Build history of the part. All positions in model axes, mm. Face numbers are marked on the shaded views. Give positions to 0.01 mm unless a question says otherwise; leave off trailing zeros. Order: outer loops, then holes, each group sorted by start corner. A loop starts at its lowest first (then second) coordinate and runs counter-clockwise, first axis right, second up. Notation, with made-up numbers: (80, 8) - (86, 8) arc R15 ccw to (86, 35) - close; hole circle Ø10 at (10, 33). An arc over 180 degrees is marked (long way). Use a Markdown table: item, result. Add a question column.
(1) Wall check: line 1 (Z direction, x = -13, y = 8); line 2 (Y direction, x = 12, z = 55); line 3 (Y direction, x = -12.5, z = 9). Give the ranges that are in metal, low to high.
(2) Slice it at A-A (x = 0). Write the cut outline in (y, z).
(3) Slice it at C-C (z = 29.5). Write the cut outline in (x, y), then the cut area to 3 significant figures.
(4) Mould opens along X. For the marked faces 1, 2 and 3 say: +X half, -X half, draft (parallel to the pull), parting line (faces both ways), or undercut.
(5) Flat gauge pins, fed straight in: pin 1 (18 mm diameter, centred on x = 6.5, y = 8.5, fed in from +Z); pin 2 (2 mm diameter, centred on y = 2, z = 31, fed in from +X) (3 decimals); pin 3 (6 mm diameter, centred on y = -9.5, z = 22, fed in from +X); pin 4 (1 mm diameter, centred on x = -3, z = 26.5, fed in from -Y). Where does each tip first touch, or does it go through?
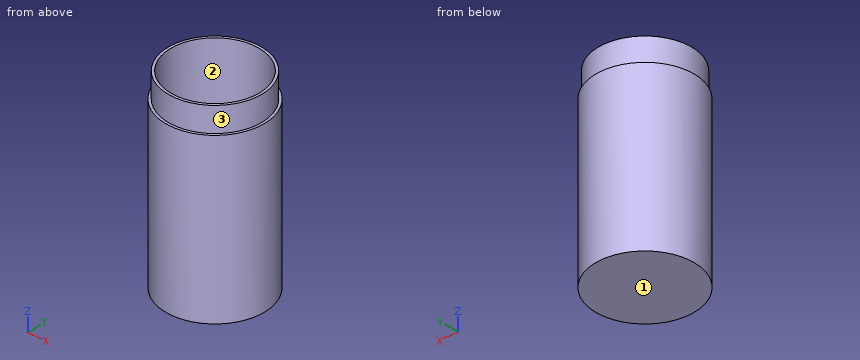
from build123d import *

# Parameters (mm, degrees)
F0_R     = 20
F1_DEPTH = 2
F2_R     = 20
F2_R_2   = 18
F3_DEPTH = 75
F4_R     = 20
F4_R_2   = 19
F5_DEPTH = 10


with BuildPart() as f1:
    # F0 (on Top) → F1 (new body)
    with BuildSketch(Plane.XY):
        Circle(F0_R)
    extrude(amount=F1_DEPTH)

    # F2 (on face) → F3 (join)
    with BuildSketch(Plane.XY.offset(2)):
        Circle(F2_R)
        Circle(F2_R_2, mode=Mode.SUBTRACT)
    extrude(amount=F3_DEPTH)

    # F4 (on face) → F5 (cut)
    with BuildSketch(Plane.XY.offset(77)):
        Circle(F4_R)
        Circle(F4_R_2, mode=Mode.SUBTRACT)
    extrude(amount=-F5_DEPTH, mode=Mode.SUBTRACT)


solid = f1.part
Solution:
| question | item | result |
|---|---|---|
| 1 | line 1 | 0 to 2 |
| 1 | line 2 | -16 to -13.42, 13.42 to 16 |
| 1 | line 3 | -15.61 to -12.95, 12.95 to 15.61 |
| 2 | outline | (-20, 0) - (20, 0) - (20, 67) - (19, 67) - (19, 77) - (18, 77) - (18, 2) - (-18, 2) - (-18, 77) - (-19, 77) - (-19, 67) - (-20, 67) - close |
| 3 | outline | circle Ø40 at (0, 0); hole circle Ø36 at (0, 0) |
| 3 | area | 239 mm2 |
| 4 | face 1 | draft |
| 4 | face 2 | undercut |
| 4 | face 3 | parting line |
| 5 | pin 1 | z = 77 |
| 5 | pin 2 | x = 19.975 |
| 5 | pin 3 | x = 18.91 |
| 5 | pin 4 | y = -19.84 |
